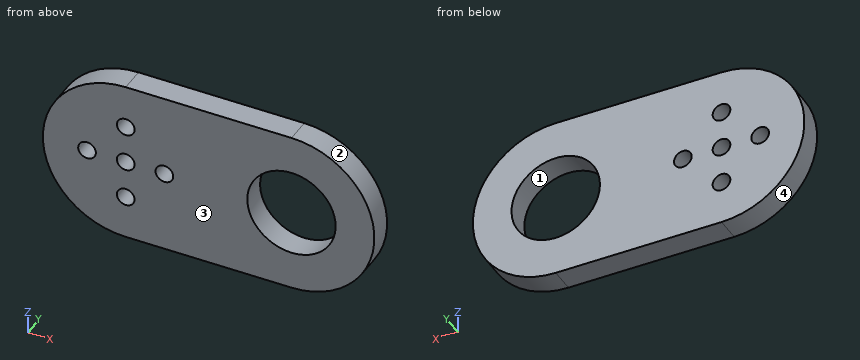
from build123d import *

# Parameters (mm, degrees)
BOSS_EXTRUDE1_DEPTH     = 4.5
SKETCH4_R               = 1.6
SERVO_HORN_HOLES_DEPTH  = 34.841542518
SKETCH5_R               = 8
BEARING_PRESS_FIT_DEPTH = 34.841542518


with BuildPart() as part:
    # Sketch2 → Boss-Extrude1 (new body)
    with BuildSketch(Plane(origin=(0, 0, 0), x_dir=(1, 0, 0), z_dir=(0, 1, 0))):
        with BuildLine():
            Line((15, 15), (-15, 15))
            ThreePointArc((-15, 15), (-30, 0), (-15, -15))
            Line((-15, -15), (15, -15))
            ThreePointArc((15, -15), (30, 0), (15, 15))
        make_face()
    extrude(amount=BOSS_EXTRUDE1_DEPTH)

    # Sketch4 → Servo horn holes (cut, through all)
    with BuildSketch(Plane(origin=(0, 4.5, 0), x_dir=(1, 0, 0), z_dir=(0, 1, 0))):
        with Locations(Location((-15, 0, 0), (0, 0, 270))):
            Circle(SKETCH4_R)
        with Locations(Location((-8, 0, 0), (0, 0, 270))):
            Circle(SKETCH4_R)
        with Locations(Location((-15, -7, 0), (0, 0, 270))):
            Circle(SKETCH4_R)
        with Locations(Location((-22, 0, 0), (0, 0, 270))):
            Circle(SKETCH4_R)
        with Locations(Location((-15, 7, 0), (0, 0, 270))):
            Circle(SKETCH4_R)
    extrude(amount=-SERVO_HORN_HOLES_DEPTH, mode=Mode.SUBTRACT)

    # Sketch5 → Bearing press fit (cut, through all)
    with BuildSketch(Plane(origin=(0, 0, 0), x_dir=(-1, 0, 0), z_dir=(0, -1, 0))):
        with Locations(Location((-15, 0, 0), (0, 0, 90))):
            Circle(SKETCH5_R)
    extrude(amount=-BEARING_PRESS_FIT_DEPTH, mode=Mode.SUBTRACT)


solid = part.part
Design review of the part built by this model. Coordinates are the model's own, in mm. Face numbers are marked on the shaded views. Give positions to 0.01 mm unless a question says otherwise; leave off trailing zeros. Loops run counter-clockwise (first coordinate to the right, second up) from the corner with the lowest first, then second, coordinate; pieces in that order, holes last. Notation, with made-up numbers: (77, -18.75) - (112, -18.75) arc R11 ccw to (112, -7.75) - close; hole circle Ø11 at (-14.5, 79). An arc over 180 degrees is marked (long way). Write item = value, one per line.
1) Take a section at A-A on y = 1.3. State the section outline as (x, z) points.
Result sheet:
outline = (-15, -15) - (15, -15) arc R15 ccw to (15, 15) - (-15, 15) arc R15 ccw to start; hole circle Ø3.2 at (-22, 0); hole circle Ø3.2 at (-15, -7); hole circle Ø3.2 at (-15, 0); hole circle Ø3.2 at (-15, 7); hole circle Ø3.2 at (-8, 0); hole circle Ø16 at (15, 0)
2) Clearance check with flat-ended pins moving along their axes: pin 1 Ø14.5 at (x, z) = (15, 0) entering from +Y; pin 2 Ø1.5 at (y, z) = (3.5, 3) entering from +X. State where each tip first meets the part, or that it passes through.
Result sheet:
pin_1 = through
pin_2 = 29.83
3) Take a section at C-C on x = -22. State the section outline as (y, z) points, and give its area (3 significant figures).
Result sheet:
outline = (0, -13.27) - (4.5, -13.27) - (4.5, -1.6) - (0, -1.6) - close; (0, 1.6) - (4.5, 1.6) - (4.5, 13.27) - (0, 13.27) - close
area = 105 mm2
4) Take a section at D-D on z = -4. State the section outline as (x, y) points, and give its area (3 significant figures).
Result sheet:
outline = (-29.46, 0) - (8.07, 0) - (8.07, 4.5) - (-29.46, 4.5) - close; (21.93, 0) - (29.46, 0) - (29.46, 4.5) - (21.93, 4.5) - close
area = 203 mm2
5) Draft analysis for pull direction X (two halves, no side actions). For the marked faces 1, 2, 3 and 4, state which applies: +X half, -X half, draft (parallel to the pull), parting line (faces both ways), or undercut.
Result sheet:
face_1 = undercut
face_2 = +X half
face_3 = draft
face_4 = -X half
6) Take a section at B-B on z = 7. State the section outline as (x, y) points.
Result sheet:
outline = (-28.27, 0) - (-16.6, 0) - (-16.6, 4.5) - (-28.27, 4.5) - close; (-13.4, 0) - (11.13, 0) - (11.13, 4.5) - (-13.4, 4.5) - close; (18.87, 0) - (28.27, 0) - (28.27, 4.5) - (18.87, 4.5) - close
7) To check wall thickness, follow line 1 (X direction, y = 2, z = 0); line 2 (Z direction, x = -14, y = 3.8); line 3 (Z direction, x = -21, y = 3.35). State the ranges of each line that lie inside material, in increasing order.
Result sheet:
line_1 = -30 to -23.6, -20.4 to -16.6, -13.4 to -9.6, -6.4 to 7, 23 to 30
line_2 = -15 to -8.25, -5.75 to -1.25, 1.25 to 5.75, 8.25 to 15
line_3 = -13.75 to -1.25, 1.25 to 13.75
